Can you work these out from the drawing? Everything is in mm from the part's minimum corner. A direction names the side the tool comes from. Round coordinates to 2 decimals unless told otherwise and drop trailing zeros. Write each loop counter-clockwise with the first axis right and the second up, starting at its lowest first coordinate (ties: lowest second). Pieces come first, ordered by that corner, then holes.
Q1. We'd pull the mould along X, two halves only. Please class the marked faces 4, 5 and 6: +X half, -X half, draft (parallel to the pull), parting line (faces both ways), or undercut.
Q2. Please list where these lines run through material, in increasing order: line 1 along X through (y, z) = (13.5, 6); line 2 along Z through (x, y) = (9.75, 18.25).
Q3. I'm going to push flat-ended pins straight in: pin 1 Ø0.9 at (x, z) = (1, 3) entering from +Y; pin 2 Ø10 at (x, z) = (9.5, 24) entering from +Y; pin 3 Ø2.5 at (y, z) = (25.5, 2.5) entering from +X; pin 4 Ø9 at (x, y) = (23.5, 22) entering from -Z. Where does each tip first touch, or does it pass through?
Q4. If we section it at A-A (x = 13.5): Please give me the cut outline in (y, z).
Q5. If we section it at B-B (y = 8.5): Please give me the cut outline in (x, z).
Q6. If we section it at C-C (z = 81.5): Please give me the cut outline in (x, y) (1 decimal).
Q7. For the marked faces 1, 2 and 3, which set-ups out of +Z, -Z, +X, -X, +Y, -Y let a thin tool reach every point of the face, with its end or its side?
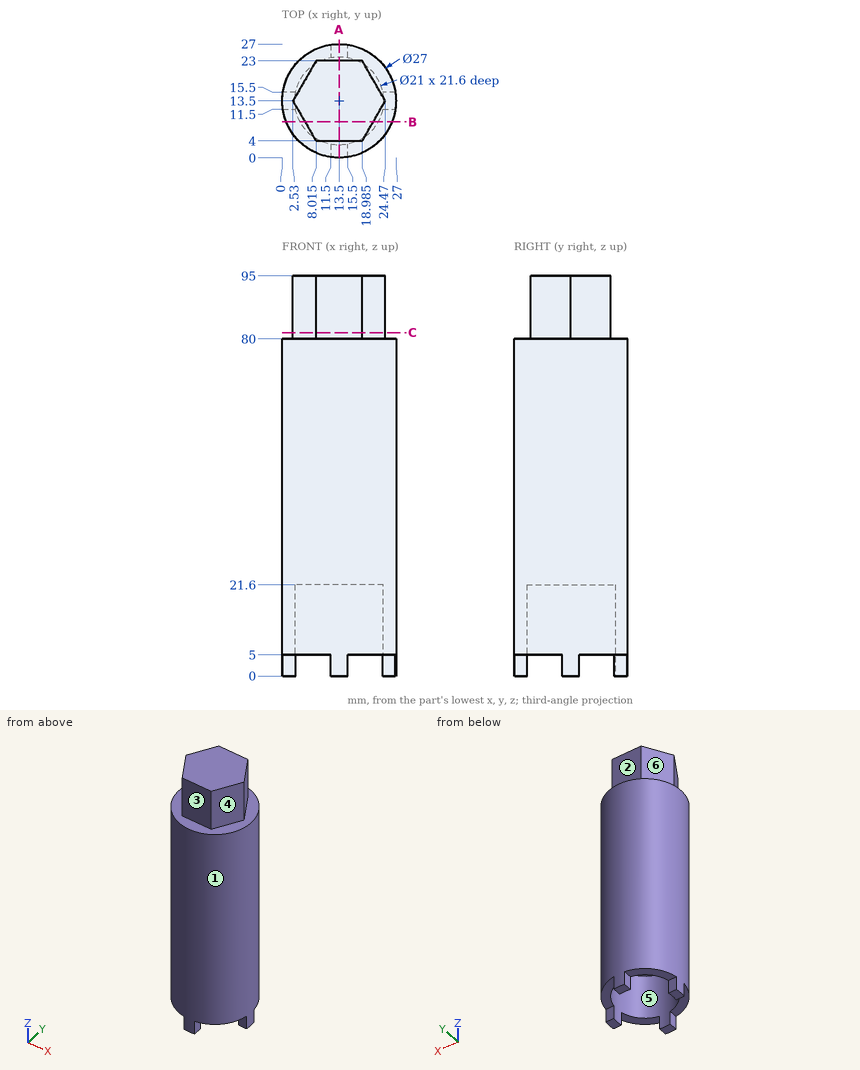
A:
1. face 4: +X half
1. face 5: undercut
1. face 6: -X half
2. line 1: x = 0 to 3, 24 to 27
2. line 2: z = 21.6 to 95
3. pin 1: stops at y = 15.5
3. pin 2: stops at y = 27
3. pin 3: stops at x = 15.5
3. pin 4: stops at z = 5
4. outline: (0, 0) - (3, 0) - (3, 21.6) - (24, 21.6) - (24, 0) - (27, 0) - (27, 80) - (23, 80) - (23, 95) - (4, 95) - (4, 80) - (0, 80) - close
5. outline: (0.96, 5) - (4.27, 5) - (4.27, 21.6) - (22.73, 21.6) - (22.73, 5) - (26.04, 5) - (26.04, 80) - (21.58, 80) - (21.58, 95) - (5.42, 95) - (5.42, 80) - (0.96, 80) - close
6. outline: (2.5, 13.5) - (8, 4) - (19, 4) - (24.5, 13.5) - (19, 23) - (8, 23) - close
7. face 1: +Z, -Z
7. face 2: +Z, +X, -X, +Y
7. face 3: +Z, +X, -X, -Y
